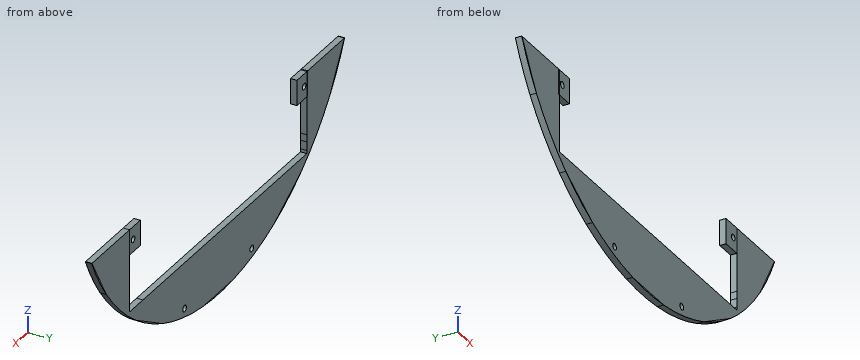
Autodesk Inventor part; units mm, degrees
ref_plane "Plano de trabajo1" through (-3.6477, -5.1016, -7.3334) normal (0, 1, 0) x (1, 0, 0)
ref_plane "Plano de trabajo2" through (-3.6477, -4.9016, -7.3334) normal (0, 1, 0) x (1, 0, 0)
ref_plane "Plano de trabajo3" through (-7.1593, -4.0366, -3.8824) normal (-1, 0, 0.0004) x (0.0004, 0, 1)
ref_plane "Plano de trabajo1" through (-3.6477, -5.1016, -7.3334) normal (0, 1, 0) x (1, 0, 0)
sketch "Boceto1" plane through (-3.6477, -5.1016, -7.3334) normal (0, 1, 0) x (1, 0, 0)
  line L0 (5.2883, -3.4507) -> (5.2882, -3.8566)
  line L1 (4.7883, -3.4507) -> (5.2883, -3.4507)
  line L2 (5.2882, -3.8566) -> (5.2882, -4.1566)
  line L3 (5.2881, -4.2507) -> (4.0881, -4.2506)
  line L4 (-3.5114, -3.8566) -> (-3.5113, -4.1566)
  line L5 (-3.5114, -3.8566) -> (-3.5116, -3.451)
  line L6 (-3.5116, -3.451) -> (-3.0116, -3.4508)
  line L7 (-3.7131, -1.2144) -> (-2.2169, -0.3506)
  line L8 (-6.2177, -4.3514) -> (-5.3539, -2.8553)
  line L9 (7.1305, -2.8553) -> (7.9943, -4.3514)
  line L10 (3.9936, -0.3506) -> (5.4897, -1.2144)
  line L11 (0.0245, 0.25) -> (1.7521, 0.25)
  arc A0 (7.9495, -4.2507) -> (-6.173, -4.251) centre (0.8883, -7.4566) ccw
  line L12 (-2.3112, -4.2505) -> (-3.5112, -4.251)
  line L13 (5.2881, -4.2507) -> (7.9495, -4.2507)
  line L14 (-3.5112, -4.251) -> (-6.173, -4.251)
  line L15 (-3.5112, -4.251) -> (-3.5116, -3.451)
  line L16 (-3.5116, -3.451) -> (5.2883, -3.4507)
  line L17 (5.2883, -3.4507) -> (5.2881, -4.2507)
  point P0 (3.6477, -7.3334)
extrude "Extrusión1" add sketch "Boceto1" along normal blind 0.2
ref_plane "Plano de trabajo2" through (-3.6477, -4.9016, -7.3334) normal (0, 1, 0) x (1, 0, 0)
sketch "Boceto2" plane through (-3.6477, -4.9016, -7.3334) normal (0, 1, 0) x (1, 0, 0)
  line L0 (5.0906, -1.7512) -> (-3.3106, -1.7469)
  line L1 (-3.3106, -1.8516) -> (-3.9207, -1.8515)
  line L2 (5.8384, -2.2498) -> (5.8385, -2.023)
  line L3 (-4.0622, -2.0234) -> (-4.0621, -2.2502)
  line L4 (5.8385, -2.023) -> (5.8385, -4.7089)
  line L5 (-4.0622, -2.0234) -> (-4.0622, -5.784)
  line L6 (5.0906, -1.7512) -> (-3.3106, -1.7469)
  line L7 (5.8385, -2.023) -> (5.8385, -1.7512)
  line L8 (5.8385, -1.7512) -> (5.0906, -1.7512)
  line L9 (-3.3106, -1.7469) -> (-4.0637, -1.7512)
  line L10 (-4.0637, -1.7512) -> (-4.0622, -2.0234)
  line L11 (5.8385, -4.7089) -> (-4.0637, -4.7089)
  line L12 (-4.0637, -4.7089) -> (-4.0637, -1.7512)
  line L13 (-4.0637, -1.7512) -> (5.8385, -1.7512)
  line L14 (5.8385, -1.7512) -> (5.8385, -4.7089)
  line L15 (5.0906, -1.6539) -> (-3.3105, -1.6519)
  line L16 (-4.0637, -1.7512) -> (5.8385, -1.7512)
  line L17 (5.8385, -1.7512) -> (5.8385, -1.654)
  line L18 (5.8385, -1.654) -> (-4.0637, -1.654)
  line L19 (-4.0637, -1.654) -> (-4.0637, -1.7512)
  point P0 (3.6477, -7.3334)
  point P1 (-3.2616, -3.4509)
extrude "Extrusión2" cut sketch "Boceto2" against normal blind 0.2
ref_plane "Plano de trabajo3" through (-7.1593, -4.0366, -3.8824) normal (-1, 0, 0.0004) x (0.0004, 0, 1)
sketch "Boceto3" plane through (-7.1593, -4.0366, -3.8824) normal (-1, 0, 0.0004) x (0.0004, 0, 1)
  line L0 (0.7998, -1.065) -> (0.7998, -0.865)
  line L1 (-1.7972, -1.065) -> (0.7998, -1.065)
  line L2 (-1.7972, -0.865) -> (-1.7972, -1.065)
  line L3 (0.7998, -0.865) -> (-1.7972, -0.865)
  line L4 (0, -1.065) -> (0, -0.4397)
  line L5 (0.7998, -0.865) -> (0, -0.865)
  line L6 (0, -0.865) -> (0, -1.065)
  line L7 (0, -1.065) -> (0.7998, -1.065)
  line L8 (0.7998, -1.065) -> (0.7998, -0.865)
  point P0 (3.8854, 4.0366)
extrude "Extrusión3" add sketch "Boceto3" along normal blind 0.6 contours L1 L4 L3 L0
ref_plane "Plano de trabajo4" through (2.1908, -4.9016, -5.3103) normal (-1, 0, 0) x (0, 0, 1)
sketch "Boceto4" plane through (2.1908, -4.9016, -5.3103) normal (-1, 0, 0) x (0, 0, 1)
  line L0 (2.2277, -0.2) -> (2.2277, 0)
  line L1 (1.4279, 0) -> (1.4279, -0.2)
  line L2 (2.2277, 0) -> (1.4279, 0)
  line L3 (1.4279, -0.2) -> (2.2277, -0.2)
  point P0 (5.3103, 4.9016)
extrude "Extrusión4" add sketch "Boceto4" along normal blind 0.6
sketch "Boceto5" plane through (-3.6477, -4.9016, -7.3334) normal (0, 1, 0) x (1, 0, 0)
  line L0 (-3.5116, -3.451) -> (-3.5112, -4.2507)
  line L1 (-3.5112, -4.2507) -> (-4.3112, -4.251)
  line L2 (-4.1112, -4.251) -> (-6.173, -4.251)
  line L3 (-3.5116, -3.451) -> (-3.5112, -4.2507)
  circle A0 centre (-3.9114, -3.851) radius 0.1
  line L4 (5.2385, -3.451) -> (5.2385, -4.2507)
  line L5 (5.2385, -3.451) -> (5.2385, -4.2507)
  line L6 (5.2385, -4.2507) -> (6.0385, -4.2507)
  line L7 (5.8385, -4.2507) -> (7.9495, -4.2507)
  line L8 (5.8385, -3.451) -> (5.2385, -3.451)
  circle A1 centre (5.6385, -3.8509) radius 0.1
  point P0 (3.6477, -7.3334)
  dimension "d9" = 0.8
  dimension "d10" = 0.2
  dimension "d11" = 0.8
  dimension "d12" = 0.2
extrude "Extrusión5" cut sketch "Boceto5" against normal blind 0.6
sketch "Boceto6" plane through (-3.6477, -5.1016, -7.3334) normal (0, -1, 0) x (1, 0, 0)
  circle A0 centre (-0.9872, 0.207) radius 0.1
  circle A1 centre (2.7638, 0.207) radius 0.1
  point P0 (3.6477, 7.3334)
extrude "Extrusión6" cut sketch "Boceto6" against normal blind 1
properties part number "va"
Work out the finished part from the listing and answer in its coordinate system (mm). Coordinates: 2 decimals unless noted, no trailing zeros. Loops run counter-clockwise (first coordinate to the right, second up) from the corner with the lowest first, then second, coordinate; pieces in that order, holes last. Notation, with made-up numbers: M -21.75,18.5 L 21.25,18.5 A27 ccw 21.25,54.5 Z; hole C 53,62 d10. An arc over 180 degrees is marked long. Use CSV: the item, a comma, the result in double quotes. Start each with the question number.
(1) Find section A-A, the plane z = -3.75. Give the vertices of the cut face in (x, y).
(2) Find section D-D, the plane z = -4.75. Give the vertices of the cut face in (x, y).
(3) Find section B-B, the plane y = -5. State how many separate pieces and enclosed holes the cut face has, then the cut area to 3 significant figures.
(4) Find section C-C, the plane x = -6.5. Give the vertices of the cut face in (y, z), then the cut area to 3 significant figures.
(5) Consider line 1 (X direction, y = -5, z = -4.4); line 2 (X direction, y = -4.95, z = -4.55); line 3 (Z direction, x = -7.25, y = -5). Determine where each line is inside the solid, lowest interval first.
Recorded:
1,outline,"M -9.48,-5.1 L -7.16,-5.1 L -7.16,-4.9 L -9.48,-4.9 Z; M 1.59,-5.1 L 3.96,-5.1 L 3.96,-4.9 L 1.59,-4.9 Z"
2,outline,"M -8.79,-5.1 L -7.71,-5.1 L -7.71,-4.9 L -8.79,-4.9 Z; M 2.19,-5.1 L 3.27,-5.1 L 3.27,-4.9 L 2.19,-4.9 Z"
3,separate pieces,"1"
3,enclosed holes,"4"
3,area,"21.3 mm^2"
4,outline,"M -5.1,-6.67 L -4.9,-6.67 L -4.9,-5.68 L -5.1,-5.68 Z"
4,area,"0.198 mm^2"
5,line 1,"x = -9.06 to -7.71, 2.19 to 3.54"
5,line 2,"x = -8.95 to -7.71, 2.19 to 3.43"
5,line 3,"z = -6.2 to -5.68, -3.88 to -3.08"
